from build123d import *

# Parameters (mm, degrees)
F0_W     = 685.8
F0_H     = 787.4
F1_DEPTH = 990.6
F2_R     = 253.930525
F3_DEPTH = 50.8
F4_R     = 50.8


with BuildPart() as f1:
    # F0 (on Top) → F1 (new body)
    with BuildSketch(Plane.XY):
        Rectangle(F0_W, F0_H)
    extrude(amount=F1_DEPTH)

    # F2 (on face) → F3 (join)
    with BuildSketch(Plane.XZ.offset(393.7)):
        with Locations((0, 532.897532)):
            Circle(F2_R)
    extrude(amount=F3_DEPTH)

    # F4
    f4_edges = [f1.edges().sort_by_distance(p)[0] for p in [
        (-342.9, -393.7, 495.3),
        (0, -393.7, 990.6),
        (342.9, -393.7, 495.3),
        (342.9, 0, 990.6),
        (0, 393.7, 990.6),
        (-342.9, 0, 990.6),
        (342.9, 393.7, 495.3),
        (342.9, 0, 0),
        (-342.9, 393.7, 495.3),
        (-342.9, 0, 0),
        (0, -393.7, 0),
        (0, 393.7, 0),
    ]]
    fillet(f4_edges, radius=F4_R)


solid = f1.part
Geometry: final body of the model. Coordinates: model frame, mm. Coordinates: 2 decimals unless noted, no trailing zeros. Order: outer loops, then holes, each group sorted by start corner. A loop starts at its lowest first (then second) coordinate and runs counter-clockwise, first axis right, second up.
1) Section C-C (x = -75). Return loops of the section in (y, z), then the cut area to 3 significant figures.
Result sheet:
outline: (-444.5, 290.3) - (-393.7, 290.3) - (-393.7, 50.8) arc R50.8 ccw to (-342.9, 0) - (342.9, 0) arc R50.8 ccw to (393.7, 50.8) - (393.7, 939.8) arc R50.8 ccw to (342.9, 990.6) - (-342.9, 990.6) arc R50.8 ccw to (-393.7, 939.8) - (-393.7, 775.5) - (-444.5, 775.5) - close
area: 802,000 mm2
2) Section A-A (x = 0). Return loops of the section in (y, z).
Result sheet:
outline: (-444.5, 278.97) - (-393.7, 278.97) - (-393.7, 50.8) arc R50.8 ccw to (-342.9, 0) - (342.9, 0) arc R50.8 ccw to (393.7, 50.8) - (393.7, 939.8) arc R50.8 ccw to (342.9, 990.6) - (-342.9, 990.6) arc R50.8 ccw to (-393.7, 939.8) - (-393.7, 786.83) - (-444.5, 786.83) - close
3) Section B-B (z = 811). Return loops of the section in (x, y).
Result sheet:
outline: (-342.9, -342.9) arc R50.8 ccw to (-292.1, -393.7) - (292.1, -393.7) arc R50.8 ccw to (342.9, -342.9) - (342.9, 342.9) arc R50.8 ccw to (292.1, 393.7) - (-292.1, 393.7) arc R50.8 ccw to (-342.9, 342.9) - close
4) Ray query, probe 1 along Y at (x, z) = (-42, 273); probe 2 along Y at (x, z) = (-242.5, 949); probe 3 along Z at (x, y) = (307.5, 116.5). Return the intervals inside material, ascending.
Result sheet:
probe 1: y = -393.7 to 393.7
probe 2: y = -392.86 to 392.86
probe 3: z = 2.39 to 988.21
5) First-contact query: P1, Ø10, axis at x = -219.5, z = 670.5, coming from the -Y side. Flat tip, straight axial feed; report the tip coordinate or a pass-through.
Result sheet:
P1: stops at y = -393.7
